Check sheet for the modelled part. Datum: model origin and axes. Units: mm. Face numbers are marked on the shaded views. A direction names the side the tool comes from. Give positions to 0.01 mm unless a question says otherwise; leave off trailing zeros. Write each loop counter-clockwise with the first axis right and the second up, starting at its lowest first coordinate (ties: lowest second). Pieces come first, ordered by that corner, then holes. Notation, with made-up numbers: (32.25, -27) -> (36.25, -27) arc R14 cw to (36.25, -23) -> close; hole circle Ø9 at (81.5, 26.5). An arc over 180 degrees is marked (long way). Return JSON: item names as keys, results as strings.
from build123d import *

# Parameters (mm, degrees)
BOSS_EXTRUDE2_DEPTH = 1.5
FILLET1_R           = 2
SKETCH1_R           = 0.63
BOSS_EXTRUDE3_DEPTH = 4.5


with BuildPart() as part:
    # Sketch2 → Boss-Extrude2 (new, symmetric)
    with BuildSketch(Plane(origin=(0, 0, 0), x_dir=(0, 0, -1), z_dir=(1, 0, 0))):
        Polygon((-6, 12.5), (-6, 9.5), (-4.5, 9.5), (-2.22, 0), (0, 0), (-3, 12.5), align=None)
    boss_extrude2 = extrude(amount=BOSS_EXTRUDE2_DEPTH, both=True)

    # Fillet1
    fillet1_edges = [part.edges().sort_by_distance(p)[0] for p in [
        (0, 12.5, 3),
    ]]
    fillet(fillet1_edges, radius=FILLET1_R)

    # Sketch1 → Boss-Extrude3 (add)
    with BuildSketch(Plane(origin=(0, 0, 0), x_dir=(1, 0, 0), z_dir=(0, 1, 0))):
        with BuildLine():
            Line((-2.2, 1.48), (2.2, 1.48))
            ThreePointArc((2.2, 1.48), (3.68, 0), (2.2, -1.48))
            Line((2.2, -1.48), (-2.2, -1.48))
            ThreePointArc((-2.2, -1.48), (-3.68, 0), (-2.2, 1.48))
        make_face()
        with Locations(Location((-2.2, 0, 0), (0, 0, 270))):
            Circle(SKETCH1_R, mode=Mode.SUBTRACT)
        with Locations(Location((2.2, 0, 0), (0, 0, 270))):
            Circle(SKETCH1_R, mode=Mode.SUBTRACT)
    extrude(amount=BOSS_EXTRUDE3_DEPTH)

    # Mirror1: Boss-Extrude2 across plane
    add(boss_extrude2.mirror(Plane.XY))


solid = part.part
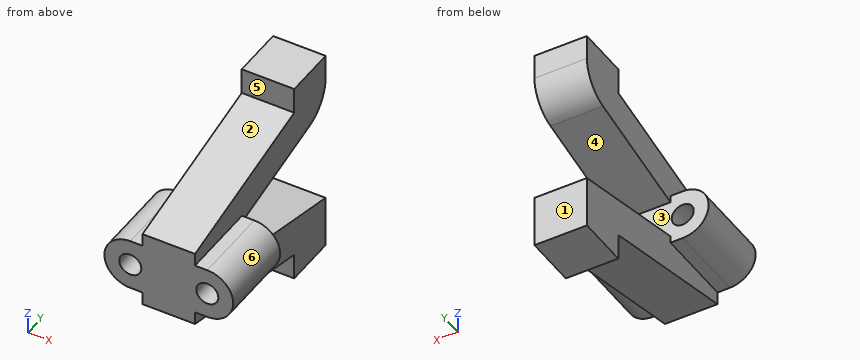
(1) Thickness scan on L1, parallel to X at y = 3.5, z = 0; L2, parallel to Y at x = -0.25, z = -1; L3, parallel to Z at x = -2.25, y = 0.5. Record the ranges inside material, lowest first.
Reply:
{"L1": "-3.68 to -2.83, -1.57 to 1.57, 2.83 to 3.68", "L2": "0 to 4.5", "L3": "-1.48 to -0.63, 0.63 to 1.48"}
(2) Cross-section at A-A on z = 0. Enter the section's corners in (x, y).
Reply:
{"outline": "(-3.68, 0) -> (-2.83, 0) -> (-2.83, 4.5) -> (-3.68, 4.5) -> close; (-1.57, 0) -> (1.57, 0) -> (1.57, 4.5) -> (-1.57, 4.5) -> close; (2.83, 0) -> (3.68, 0) -> (3.68, 4.5) -> (2.83, 4.5) -> close"}
(3) Depth check by flat-ended pin: pin 1 Ø1.5 at (y, z) = (6.5, 3) entering from -X; pin 2 Ø4 at (y, z) = (5, 3) entering from +X; pin 3 Ø0.9 at (x, z) = (-1.5, 0.5) entering from +Y; pin 4 Ø1.1 at (x, z) = (-2.2, 0) entering from -Y. Enter the tip coordinate at first touch or a pass-through.
Reply:
{"pin 1": "x = -1.5", "pin 2": "x = 3.23", "pin 3": "y = 4.5", "pin 4": "through"}
(4) Cross-section at B-B on y = 2.5. Enter the section's corners in (x, z).
Reply:
{"outline": "(-2.2, -1.48) -> (-1.5, -1.48) -> (-1.5, -2.82) -> (1.5, -2.82) -> (1.5, -1.48) -> (2.2, -1.48) arc R1.48 ccw to (2.2, 1.48) -> (1.5, 1.48) -> (1.5, 2.82) -> (-1.5, 2.82) -> (-1.5, 1.48) -> (-2.2, 1.48) arc R1.48 ccw to start; hole circle Ø1.26 at (-2.2, 0); hole circle Ø1.26 at (2.2, 0)"}
(5) Cross-section at C-C on y = 6.75. Enter the section's corners in (x, z), then the cut area to 3 significant figures.
Reply:
{"outline": "(-1.5, -3.84) -> (1.5, -3.84) -> (1.5, -1.62) -> (-1.5, -1.62) -> close; (-1.5, 1.62) -> (1.5, 1.62) -> (1.5, 3.84) -> (-1.5, 3.84) -> close", "area": "13.3 mm^2"}
(6) Set-up check for the marked faces 4, 5 and 6: record each of +Z, -Z, +X, -X, +Y, -Y from which the full face is reachable in a straight line by a thin tool's end or side.
Reply:
{"face 4": "+X, -X, +Y", "face 5": "+Z, +X, -X, -Y", "face 6": "+X, +Y, -Y"}
(7) Cross-section at D-D on x = -0.25. Enter the section's corners in (y, z), then the cut area to 3 significant figures.
Reply:
{"outline": "(0, -2.22) -> (9.5, -4.5) -> (9.5, -6) -> (12.5, -6) -> (12.5, -3) -> (4.5, -1.08) -> (4.5, 1.08) -> (10.97, 2.63) arc R2 ccw to (12.5, 4.58) -> (12.5, 6) -> (9.5, 6) -> (9.5, 4.5) -> (0, 2.22) -> close", "area": "66.7 mm^2"}
(8) Release check for a two-part mould opening along Z. For the marked faces 1, 2 and 3 record: pulls with the +Z half, pulls with the -Z half, needs draft (parallel to the pull), parting line crosses it, or undercut.
Reply:
{"face 1": "needs draft", "face 2": "pulls with the +Z half", "face 3": "undercut"}
